Autodesk Inventor part; units mm, degrees
ref_plane "YZ Plane" through (0, 0, 0) normal (1, 0, 0) x (0, 1, 0)
ref_plane "XZ Plane" through (0, 0, 0) normal (0, 1, 0) x (-1, 0, 0)
ref_plane "XY Plane" through (0, 0, 0) normal (0, 0, 1) x (1, 0, 0)
ref_plane "Work Plane1" through (8.001, 26.0985, -18.0717) normal (0, 1, 0) x (0, 0, -1)
sketch "Sketch1" plane through (8.001, 26.0985, -18.0717) normal (0, 1, 0) x (0, 0, -1)
  line L0 (-43.7282, -1.4601) -> (-43.7282, -1.8842)
  line L1 (-43.7282, -1.8842) -> (-9.3098, -1.8842)
  line L2 (-9.3098, -1.8842) -> (-9.3098, 2.815)
  line L3 (-43.7282, 11.0271) -> (-43.7282, 11.4512)
  line L4 (-43.7282, 11.4512) -> (-9.3098, 11.4512)
  line L5 (-9.3098, 11.4512) -> (-9.3098, 6.752)
  line L6 (-43.7282, -1.4601) -> (-43.7282, 11.0271)
  line L7 (-9.3098, 2.815) -> (-25.0363, 2.815)
  line L8 (-25.0363, 2.815) -> (-25.0363, 6.752)
  line L9 (-25.0363, 6.752) -> (-9.3098, 6.752)
  line L10 (-18.0537, 2.815) -> (-18.0537, -1.8842) construction
  line L11 (-18.0537, 6.752) -> (-18.0537, 11.4512) construction
  line L12 (-16.6851, 3.45) -> (-16.6851, 6.117) construction
  line L13 (-16.6851, 3.45) -> (-12.9069, 3.45) construction
  line L14 (-12.9069, 3.45) -> (-12.9069, 6.117) construction
  line L15 (-12.9069, 6.117) -> (-16.6851, 6.117) construction
  point P0 (-18.0717, 8.001)
  dimension "d19" = 0.635
  dimension "d20" = 0.635
extrude "Extrusion1" add sketch "Sketch1" along normal blind 7.9375
sketch "Sketch2" plane through (9.8852, 26.0985, 25.6565) normal (1, 0, 0) x (0, 0, -1)
  line L0 (34.4184, 0) -> (0, 0) construction
  line L1 (34.4184, 0) -> (34.4184, 7.9375) construction
  line L2 (0, 7.9375) -> (34.4184, 7.9375) construction
  line L3 (0, 0) -> (0, 7.9375) construction
  line L4 (34.4184, 0) -> (34.4184, 7.9375) construction
  line L5 (34.4184, 3.9687) -> (0, 3.9687) construction
  line L6 (34.4184, 0) -> (0, 0) construction
  line L7 (28.9311, 0) -> (28.9311, 7.9375) construction
  line L8 (34.4184, 7.9375) -> (14.8298, 7.9375) construction
  circle A0 centre (28.9311, 3.9687) radius 1.9304
  point P0 (25.6565, -26.0985)
  dimension "d8" = 3.8608
extrude "Extrusion2" cut sketch "Sketch2" against normal through all
fillet "Fillet1" radius 3.175 2 edges at (3.2175, 34.036, 25.6565) (3.2175, 26.0985, 25.6565)
sketch "Sketch3" plane through (9.8852, 26.0985, -8.7619) normal (1, 0, 0) x (0, 0, -1)
  circle A0 centre (-5.4873, 3.9688) radius 1.9304
  line L0 (0, 0) -> (-31.2434, 0)
  line L1 (0, 0) -> (0, 7.9375)
  line L2 (-31.2434, 7.9375) -> (0, 7.9375)
  line L3 (-34.4184, 3.175) -> (-34.4184, 4.7625)
  line L4 (-31.2434, 3.175) -> (-31.2434, 4.7625) construction
  circle A1 centre (-31.2434, 3.9687) radius 1.7859
  arc A2 (-34.4184, 3.175) -> (-31.2434, 0) centre (-31.2434, 3.175) ccw
  arc A3 (-31.2434, 7.9375) -> (-34.4184, 4.7625) centre (-31.2434, 4.7625) ccw
  point P0 (-8.7619, -26.0985)
  dimension "d7" = 3.5719
extrude "Extrusion3" cut sketch "Sketch3" against normal through all contours A1
sketch "Sketch5" plane through (9.8852, 26.0985, -8.7619) normal (1, 0, 0) x (0, 0, -1)
  circle A0 centre (-31.2434, 3.9688) radius 1.7859 construction
  circle A1 centre (-5.4873, 3.9688) radius 1.9304 construction
  line L0 (0, 0) -> (-31.2434, 0) construction
  line L1 (0, 0) -> (0, 7.9375) construction
  line L2 (-31.2434, 7.9375) -> (0, 7.9375) construction
  line L3 (-34.4184, 3.175) -> (-34.4184, 4.7625) construction
  line L4 (-15.9544, 0) -> (0, 0)
  line L5 (-2.2351, 0) -> (-2.2351, 7.9375)
  line L6 (-15.9544, 7.9375) -> (0, 7.9375)
  line L7 (-2.2351, 0) -> (-8.7527, 0)
  line L8 (-34.4184, 7.9375) -> (0, 7.9375)
  line L9 (-2.2351, 0) -> (0, 0)
  line L10 (0, 0) -> (0, 7.9375)
  line L11 (0, 7.9375) -> (-2.2351, 7.9375)
  line L12 (-2.2351, 7.9375) -> (-2.2351, 0)
  arc A2 (-34.4184, 3.175) -> (-31.2434, 0) centre (-31.2434, 3.175) ccw
  arc A3 (-31.2434, 7.9375) -> (-34.4184, 4.7625) centre (-31.2434, 4.7625) ccw
  point P0 (-8.7619, -26.0985)
extrude "Extrusion4" cut sketch "Sketch5" against normal through all
fillet "Fillet2" radius 3.175 4 edges at (7.5356, 34.036, -6.5269) (-1.1006, 34.036, -6.5269) (7.5356, 26.0985, -6.5269) (-1.1006, 26.0985, -6.5269)
sketch "Sketch6" plane through (8.001, 26.0985, -18.0717) normal (0, -1, 0) x (1, 0, 0)
  line L0 (-1.7153, 46.6729) -> (-1.7153, 39.3669) construction
  line L1 (-8.0653, 39.3669) -> (-8.0653, 46.6729) construction
  line L2 (-1.0803, 47.2656) -> (-1.0803, 39.3486) construction
  line L3 (-8.7003, 39.3486) -> (-8.7003, 42.6343) construction
  line L4 (-1.0803, 47.2656) -> (-8.7003, 47.2656)
  line L5 (-8.7003, 47.2656) -> (-8.7003, 31.0791)
  line L6 (-8.7003, 31.0791) -> (-1.0803, 31.0791)
  line L7 (-1.0803, 31.0791) -> (-1.0803, 47.2656)
  point P0 (-8.001, 18.0717)
  dimension "d12" = 0.635
  dimension "d13" = 0.635
extrude "Extrusion5" cut sketch "Sketch6" against normal through all
sketch "Sketch8" plane through (-3.4502, 29.2735, 25.6565) normal (-1, 0, 0) x (0, 0, 1)
  arc A0 (-32.1833, 0) -> (-29.0083, -3.175) centre (-29.0083, 0) ccw construction
  line L0 (-3.175, -3.175) -> (-29.0083, -3.175) construction
  arc A1 (-3.175, -3.175) -> (0, 0) centre (-3.175, 0) ccw construction
  line L1 (0, 0) -> (0, 1.5875) construction
  arc A2 (0, 1.5875) -> (-3.175, 4.7625) centre (-3.175, 1.5875) ccw construction
  line L2 (-29.0083, 4.7625) -> (-3.175, 4.7625) construction
  arc A3 (-29.0083, 4.7625) -> (-32.1833, 1.5875) centre (-29.0083, 1.5875) ccw construction
  line L3 (-32.1833, 1.5875) -> (-32.1833, 0) construction
  circle A4 centre (-3.175, 0.7938) radius 1.7859 construction
  circle A5 centre (-28.9311, 0.7938) radius 1.9304 construction
  line L4 (-3.175, 4.7625) -> (-29.0083, 4.7625)
  line L5 (-6.2153, 4.7625) -> (-16.0917, 4.7625)
  line L6 (-16.0917, 4.7625) -> (-16.0917, 3.1144)
  line L7 (-16.0917, 3.1144) -> (-6.2153, 3.1144)
  line L8 (-6.2153, 3.1144) -> (-6.2153, 4.7625)
  point P0 (-25.6565, -29.2735)
extrude "Extrusion7" add sketch "Sketch8" along normal blind 6.35
fillet "Fillet3" radius 3.175 1 edges at (-3.4502, 32.3879, 14.503)
properties part number "lever2"
Could you check a few things on this model? Use its own coordinates, in mm. A direction names the side the tool comes from. Give positions to 0.01 mm unless a question says otherwise; leave off trailing zeros. Order: outer loops, then holes, each group sorted by start corner. A loop starts at its lowest first (then second) coordinate and runs counter-clockwise, first axis right, second up. Notation, with made-up numbers: (-29, 9) -> (-4, 9) arc R19 cw to (-4, 33) -> close; hole circle Ø2 at (66.5, 63). An arc over 180 degrees is marked (long way). Answer in a Markdown table with one row per item. Add a question column.
Item 1: Please list where these lines run through material, in increasing order: probe 1 along X at (y, z) = (33.25, 1); probe 2 along X at (y, z) = (27.25, 14); probe 3 along Z at (x, y) = (5, 32.5).
Item 2: Imagine slicing it at B-B (z = -4). List the corners of the cut face in (x, y) for me.
Item 3: For faces 4 (the flat face through (3, 30, 13.007)), 5 (the flat face through (1.249, 30, 0)), 6 (the flat face through (-1, 30, -6.527)), which set-ups out of +Z, -Z, +X, -X, +Y, -Y let a thin tool reach every point of the face, with its end or its side?
Item 4: Imagine slicing it at C-C (y = 30.5). Count the separate pieces of the cut face and the enclosed holes in it, and give its area (3 significant figures).
Item 5: Imagine slicing it at A-A (z = 0). List the corners of the cut face in (x, y) for me.
Item 6: I'm going to push flat-ended pins straight in: P1, Ø4, axis at x = -7, y = 30.5, coming from the +Z side; P2, Ø1, axis at x = -8, z = 14, coming from the -Y side. Where does each tip first touch, or does it pass through?
Item 7: We'd pull the mould along X, two halves only. Please class faces 1 (the flat face through (6.921, 30, 19)), 2 (the cylindrical face through (-1.07, 31.98, -3.02)), 3 (the flat face through (-9.8, 33, 14)): pulls with the +X half, pulls with the -X half, needs draft (parallel to the pull), parting line crosses it, or undercut.
Result:
| question | item | result |
|---|---|---|
| 1 | probe 1 | -3.45 to 1.25, 5.19 to 9.89 |
| 1 | probe 2 | -3.45 to -0.7, 6.92 to 9.89 |
| 1 | probe 3 | 6.96 to 13.01 |
| 2 | outline | (-3.45, 26.17) -> (1.25, 26.17) -> (1.25, 28.28) -> (-3.45, 28.28) -> close; (-3.45, 31.86) -> (1.25, 31.86) -> (1.25, 33.97) -> (-3.45, 33.97) -> close; (5.19, 26.17) -> (9.89, 26.17) -> (9.89, 28.28) -> (5.19, 28.28) -> close; (5.19, 31.86) -> (9.89, 31.86) -> (9.89, 33.97) -> (5.19, 33.97) -> close |
| 3 | face 4 | +Z, +Y, -Y |
| 3 | face 5 | -Z, +Y, -Y |
| 3 | face 6 | -Z, +X, -X, +Y, -Y |
| 4 | separate pieces | 5 |
| 4 | enclosed holes | 0 |
| 4 | area | 227 mm2 |
| 5 | outline | (-3.45, 26.1) -> (1.25, 26.1) -> (1.25, 34.04) -> (-3.45, 34.04) -> close; (5.19, 26.1) -> (9.89, 26.1) -> (9.89, 34.04) -> (5.19, 34.04) -> close |
| 6 | P1 | z = 19.44 |
| 6 | P2 | y = 32.39 |
| 7 | face 1 | undercut |
| 7 | face 2 | needs draft |
| 7 | face 3 | pulls with the -X half |
